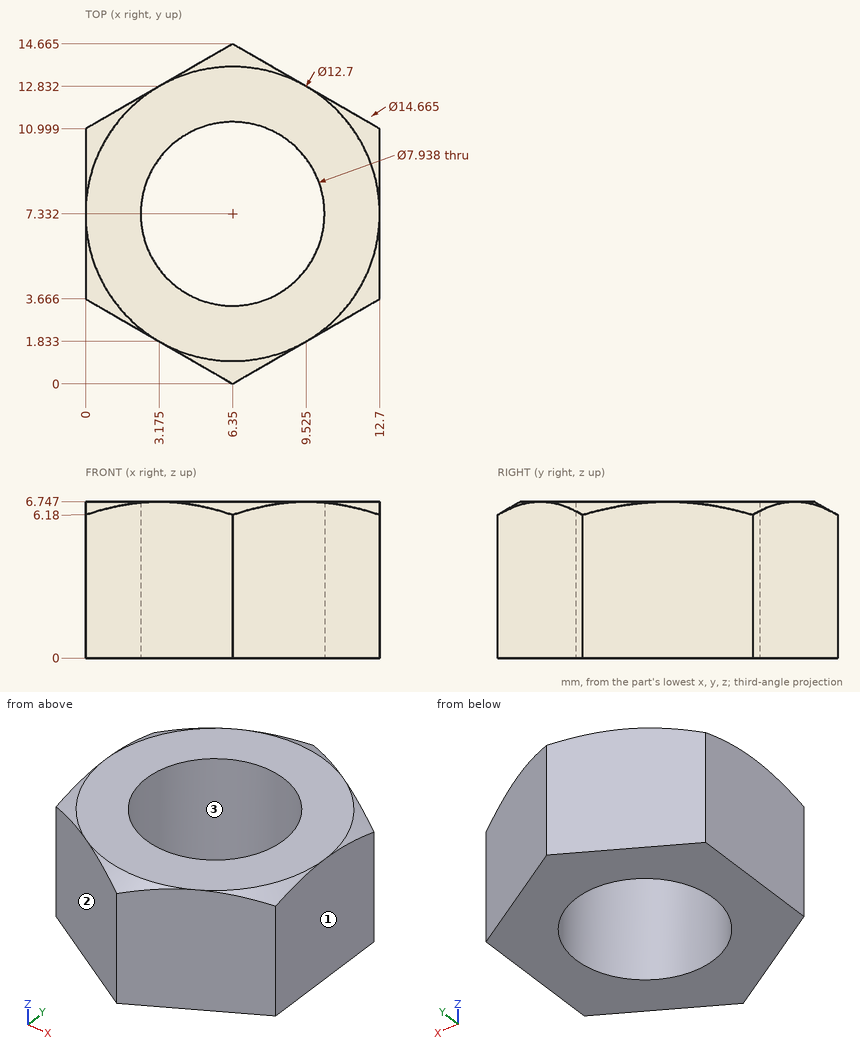
Source: three-view drawing plus pictorial views. Frame: mm from the lowest corner of the part. Round coordinates to 2 decimals unless told otherwise and drop trailing zeros. Answer in a Markdown table with one row per item.
Item 1: Mould query, pull axis X, two halves, no side actions, for the marked faces 1, 2 and 3. Classes: released by +X, released by -X, zero draft, split by the parting line, or undercut.
Model answer:
| item | result |
|---|---|
| face 1 | released by +X |
| face 2 | released by -X |
| face 3 | undercut |
Item 2: Line query: line 1 (X direction, y = 9, z = 4.5); line 2 (Y direction, x = 8.5, z = 4.5) (1 decimal); line 3 (Y direction, x = 3, z = 0.75) (1 decimal). Output: solid intervals per line, ascending.
Model answer:
| item | result |
|---|---|
| line 1 | x = 0 to 2.75, 9.95 to 12.7 |
| line 2 | y = 1.2 to 4, 10.7 to 13.4 |
| line 3 | y = 1.9 to 5.2, 9.5 to 12.7 |
Item 3: Pin query (flat end, axial travel): pin 1 (3 mm diameter, centred on x = 4.5, y = 10.5, fed in from -Z); pin 2 (1.5 mm diameter, centred on y = 2, z = 1, fed in from -X) (1 decimal); pin 3 (3 mm diameter, centred on y = 2, z = 2.5, fed in from +X) (1 decimal); pin 4 (4 mm diameter, centred on x = 4.5, z = 2, fed in from -Y). Return the tip coordinate at first contact, or that it passes through.
Model answer:
| item | result |
|---|---|
| pin 1 | stops at z = 0 |
| pin 2 | stops at x = 1.6 |
| pin 3 | stops at x = 12.4 |
| pin 4 | stops at y = 0 |
